Could you check a few things on this model? Use its own coordinates, in mm. A direction names the side the tool comes from. Coordinates: 2 decimals unless noted, no trailing zeros. Loops run counter-clockwise (first coordinate to the right, second up) from the corner with the lowest first, then second, coordinate; pieces in that order, holes last.
from build123d import *

# Parameters (mm, degrees)
SKETCH2_R           = 1.6
SKETCH2_R_2         = 4
BOSS_EXTRUDE1_DEPTH = 2


with BuildPart() as part:
    # Sketch2 → Boss-Extrude1 (new body)
    with BuildSketch(Plane(origin=(0, 0, 70.507785861), x_dir=(-1, 0, 0), z_dir=(0, 0, -1))):
        with BuildLine():
            Line((-93.581832429, -113.483945735), (-76.752691037, -96.654804343))
            ThreePointArc((-76.752691037, -96.654804343), (-73.924263912, -95.483231467), (-71.095836788, -96.654804343))
            Line((-71.095836788, -96.654804343), (-41.093354786, -126.657286344))
            ThreePointArc((-41.093354786, -126.657286344), (-38.264927661, -127.828859219), (-35.436500537, -126.657286344))
            Line((-35.436500537, -126.657286344), (-31.759545275, -122.980331082))
            ThreePointArc((-31.759545275, -122.980331082), (-30.587972399, -120.151903957), (-31.759545275, -117.323476832))
            Line((-31.759545275, -117.323476832), (-50.448318777, -98.63470333))
            ThreePointArc((-50.448318777, -98.63470333), (-51.619891652, -95.806276205), (-50.448318777, -92.97784908))
            Line((-50.448318777, -92.97784908), (-44.791464528, -87.320994831))
            ThreePointArc((-44.791464528, -87.320994831), (-43.619891652, -84.492567706), (-44.791464528, -81.664140581))
            Line((-44.791464528, -81.664140581), (-50.448318777, -76.007286332))
            ThreePointArc((-50.448318777, -76.007286332), (-51.619891652, -73.178859207), (-50.448318777, -70.350432082))
            Line((-50.448318777, -70.350432082), (-35.599076372, -55.501189677))
            ThreePointArc((-35.599076372, -55.501189677), (-34.427503497, -52.672762553), (-35.599076372, -49.844335428))
            Line((-35.599076372, -49.844335428), (-36.518315188, -48.925096612))
            ThreePointArc((-36.518315188, -48.925096612), (-37.689888063, -46.096669488), (-36.518315188, -43.268242363))
            Line((-36.518315188, -43.268242363), (-22.425735763, -29.175662938))
            ThreePointArc((-22.425735763, -29.175662938), (-21.254162888, -26.347235813), (-22.425735763, -23.518808689))
            Line((-22.425735763, -23.518808689), (-26.102691025, -19.841853427))
            ThreePointArc((-26.102691025, -19.841853427), (-28.93111815, -18.670280551), (-31.759545275, -19.841853427))
            Line((-31.759545275, -19.841853427), (-45.852124699, -33.934432851))
            ThreePointArc((-45.852124699, -33.934432851), (-48.680551824, -35.106005727), (-51.508978949, -33.934432851))
            Line((-51.508978949, -33.934432851), (-61.762027276, -23.681384524))
            ThreePointArc((-61.762027276, -23.681384524), (-64.590454401, -22.509811649), (-67.418881525, -23.681384524))
            Line((-67.418881525, -23.681384524), (-84.248022918, -40.510525916))
            ThreePointArc((-84.248022918, -40.510525916), (-87.076450042, -41.682098792), (-89.904877167, -40.510525916))
            Line((-89.904877167, -40.510525916), (-119.907359169, -10.508043915))
            ThreePointArc((-119.907359169, -10.508043915), (-122.735786293, -9.33647104), (-125.564213418, -10.508043915))
            Line((-125.564213418, -10.508043915), (-129.24116868, -14.184999177))
            ThreePointArc((-129.24116868, -14.184999177), (-130.412741556, -17.013426302), (-129.24116868, -19.841853427))
            Line((-129.24116868, -19.841853427), (-99.238686679, -49.844335428))
            ThreePointArc((-99.238686679, -49.844335428), (-98.067113804, -52.672762553), (-99.238686679, -55.501189677))
            Line((-99.238686679, -55.501189677), (-125.401637583, -81.664140581))
            ThreePointArc((-125.401637583, -81.664140581), (-126.573210458, -84.492567706), (-125.401637583, -87.320994831))
            Line((-125.401637583, -87.320994831), (-124.482398767, -88.240233646))
            ThreePointArc((-124.482398767, -88.240233646), (-123.310825892, -91.068660771), (-124.482398767, -93.897087896))
            Line((-124.482398767, -93.897087896), (-138.574978192, -107.989667321))
            ThreePointArc((-138.574978192, -107.989667321), (-139.746551067, -110.818094445), (-138.574978192, -113.64652157))
            Line((-138.574978192, -113.64652157), (-134.89802293, -117.323476832))
            ThreePointArc((-134.89802293, -117.323476832), (-132.069595805, -118.495049708), (-129.24116868, -117.323476832))
            Line((-129.24116868, -117.323476832), (-115.148589256, -103.230897408))
            ThreePointArc((-115.148589256, -103.230897408), (-112.320162131, -102.059324532), (-109.491735006, -103.230897408))
            Line((-109.491735006, -103.230897408), (-99.238686679, -113.483945735))
            ThreePointArc((-99.238686679, -113.483945735), (-96.410259554, -114.65551861), (-93.581832429, -113.483945735))
        make_face()
        with Locations((-132.055025121, -110.832665129)):
            Circle(SKETCH2_R, mode=Mode.SUBTRACT)
        with Locations((-28.945688834, -26.332665129)):
            Circle(SKETCH2_R, mode=Mode.SUBTRACT)
        with Locations((-122.750356977, -17.027996986)):
            Circle(SKETCH2_R, mode=Mode.SUBTRACT)
        with Locations((-38.250356977, -120.137333273)):
            Circle(SKETCH2_R, mode=Mode.SUBTRACT)
        with Locations((-53.276745902, -84.492567706)):
            Circle(SKETCH2_R_2, mode=Mode.SUBTRACT)
        with BuildLine():
            Line((-109.491735006, -81.664140581), (-67.418881525, -39.591287101))
            ThreePointArc((-67.418881525, -39.591287101), (-64.590454401, -38.419714226), (-61.762027276, -39.591287101))
            Line((-61.762027276, -39.591287101), (-51.508978949, -49.844335428))
            ThreePointArc((-51.508978949, -49.844335428), (-50.337406074, -52.672762553), (-51.508978949, -55.501189677))
            Line((-51.508978949, -55.501189677), (-93.581832429, -97.574043158))
            ThreePointArc((-93.581832429, -97.574043158), (-96.410259554, -98.745616033), (-99.238686679, -97.574043158))
            Line((-99.238686679, -97.574043158), (-109.491735006, -87.320994831))
            ThreePointArc((-109.491735006, -87.320994831), (-110.663307881, -84.492567706), (-109.491735006, -81.664140581))
        make_face(mode=Mode.SUBTRACT)
    extrude(amount=BOSS_EXTRUDE1_DEPTH)


solid = part.part
(1) Which directions (+Z, -Z, +X, -X, +Y, -Y) give clear straight access to the entire face, cutting with the end or side of a thin tool? Please do faces 4 (the face through (75.72, -31.98, 69.52)), 5 (the face through (88.75, -60.92, 69.52)), 6 (the face through (112.14, -68.4, 69.52)), 7 (the face through (47.58, -78.875, 69.522)).
Answers:
face 4: +Z, -Z, +Y
face 5: +Z, -Z
face 6: +Z, -Z, +X
face 7: +Z, -Z, -X
(2) Imagine slicing it at B-B, the plane x = 117.5. Write out the boundary of the cut face in (y, z), and give its area (3 significant figures).
Answers:
outline: (-105.58, 68.51) - (-73.76, 68.51) - (-73.76, 70.51) - (-105.58, 70.51) - close; (-31.58, 68.51) - (-12.92, 68.51) - (-12.92, 70.51) - (-31.58, 70.51) - close
area: 101 mm2
(3) We'd pull the mould along Y, two halves only. Please class faces 1 (the face through (131.43, -100.845, 69.522)), 2 (the face through (38.71, -26.79, 69.52)), 3 (the face through (33.62, -124.84, 69.52)): +Y half, -Y half, draft (parallel to the pull), parting line (faces both ways), or undercut.
Answers:
face 1: undercut
face 2: +Y half
face 3: -Y half
(4) Imagine slicing it at C-C, the plane z = 69.8. State how many separate pieces and enclosed holes the cut face has, and give its area (3 significant figures).
Answers:
separate pieces: 1
enclosed holes: 6
area: 4,770 mm2
(5) I need wall thicknesses on probe 1 along Y at (x, z) = (110, 70.3); probe 2 along X at (y, z) = (-111.5, 69.4); probe 3 along X at (y, z) = (-82, 70.25). Which ranges of each line are inside material? Lowest first, please.
Answers:
probe 1: y = -102.8 to -86.7, -82.29 to -66.26, -39.08 to -20.42
probe 2: x = 37.58 to 56.25, 91.6 to 101.22, 123.42 to 130.6, 133.51 to 139.69
probe 3: x = 44.49 to 50.15, 56.41 to 78.01, 109.79 to 125.7
(6) Imagine slicing it at A-A, the plane y = -67.5. Write out the boundary of the cut face in (x, z).
Answers:
outline: (47.6, 68.51) - (63.51, 68.51) - (63.51, 70.51) - (47.6, 70.51) - close; (95.33, 68.51) - (111.24, 68.51) - (111.24, 70.51) - (95.33, 70.51) - close
